Here's how the part is built. I have some questions about the finished solid (model axes, mm). A direction names the side the tool comes from. Round coordinates to 2 decimals unless told otherwise and drop trailing zeros. Loops run counter-clockwise (first coordinate to the right, second up) from the corner with the lowest first, then second, coordinate; pieces in that order, holes last. Notation, with made-up numbers: M 52.25,10.25 L 104.25,10.25 A17 ccw 104.25,33.25 Z; hole C 28,34.5 d2. An arc over 180 degrees is marked long. Use a Markdown table: item, result.
```python
from build123d import *

# Parameters (mm, degrees)
SKETCH2_R           = 41.5
SKETCH2_R_2         = 36.5
BOSS_EXTRUDE2_DEPTH = 140
BOSS_EXTRUDE3_START = -5
SKETCH13_R          = 41.5
SKETCH13_R_2        = 4.5
BOSS_EXTRUDE3_DEPTH = 5
CUT_EXTRUDE1_DEPTH  = 39
CUT_EXTRUDE2_DEPTH  = 39
CUT_EXTRUDE3_DEPTH  = 39
CUT_EXTRUDE4_DEPTH  = 39


with BuildPart() as part:
    # Sketch2 → Boss-Extrude2 (new body)
    with BuildSketch(Plane.XY):
        Circle(SKETCH2_R)
        Circle(SKETCH2_R_2, mode=Mode.SUBTRACT)
    extrude(amount=BOSS_EXTRUDE2_DEPTH)

    # Sketch13 → Boss-Extrude3 (add)
    with BuildSketch(Plane.XY.offset(BOSS_EXTRUDE3_START)):
        Circle(SKETCH13_R)
        Circle(SKETCH13_R_2, mode=Mode.SUBTRACT)
    extrude(amount=BOSS_EXTRUDE3_DEPTH)

    # Sketch14 → Cut-Extrude1 (cut)
    with BuildSketch(Plane(origin=(0, 0, 0), x_dir=(1, 0, 0), z_dir=(0, 1, 0))):
        Polygon((3.5, -127), (10.5, -127), (10.5, -122), (-3.5, -122), (-3.5, -140), (3.5, -140), align=None)
    extrude(amount=-CUT_EXTRUDE1_DEPTH, mode=Mode.SUBTRACT)

    # Sketch16 → Cut-Extrude2 (cut)
    with BuildSketch(Plane(origin=(0, 0, 0), x_dir=(0, 0, -1), z_dir=(1, 0, 0))):
        Polygon((-140, 3.548648678), (-127, 3.548648678), (-127, 10.548648678), (-122, 10.548648678), (-122, -3.451351322), (-140, -3.451351322), align=None)
    extrude(amount=CUT_EXTRUDE2_DEPTH, mode=Mode.SUBTRACT)

    # Sketch19 → Cut-Extrude3 (cut)
    with BuildSketch(Plane(origin=(0, 0, 0), x_dir=(1, 0, 0), z_dir=(0, 1, 0))):
        Polygon((3.5, -140), (3.5, -122), (-10.5, -122), (-10.5, -127), (-3.5, -127), (-3.5, -140), align=None)
    extrude(amount=CUT_EXTRUDE3_DEPTH, mode=Mode.SUBTRACT)

    # Sketch20 → Cut-Extrude4 (cut)
    with BuildSketch(Plane(origin=(0, 0, 0), x_dir=(0, 0, -1), z_dir=(1, 0, 0))):
        Polygon((-127, -3.5), (-140, -3.5), (-140, 3.5), (-122, 3.5), (-122, -10.5), (-127, -10.5), align=None)
    extrude(amount=-CUT_EXTRUDE4_DEPTH, mode=Mode.SUBTRACT)


solid = part.part
```
Q1. Will these pins go through, and if not, where does the flat tip stop? P1, Ø2, axis at x = -29, z = 95.5, coming from the -Y side; P2, Ø2, axis at y = 7, z = 94, coming from the +X side; P3, Ø6, axis at x = 16.5, y = -8, coming from the +Z side.
Return value:
| item | result |
|---|---|
| P1 | stops at y = -30.63 |
| P2 | stops at x = 41.06 |
| P3 | stops at z = 0 |
Q2. For faces 4 (the cylindrical face through (34.814, 10.964, 69.02)), 5 (the flat face through (-1, -9, -5)), 6 (the flat face through (10.5, -37, 125)), which set-ups out of +Z, -Z, +X, -X, +Y, -Y let a thin tool reach every point of the face, with its end or its side?
Return value:
| item | result |
|---|---|
| face 4 | +Z |
| face 5 | -Z, +X, -X, +Y, -Y |
| face 6 | none |
Q3. We'd pull the mould along X, two halves only. Please class faces 1 (the flat face through (24, 28, 140)), 2 (the flat face through (2, -39, 129)), 3 (the cylindrical face through (39.584, 12.465, 66.485)): pulls with the +X half, pulls with the -X half, needs draft (parallel to the pull), parting line crosses it, or undercut.
Return value:
| item | result |
|---|---|
| face 1 | needs draft |
| face 2 | undercut |
| face 3 | parting line crosses it |
Q4. I need wall thicknesses on line 1 (Y direction, x = 0, z = 67); line 2 (Z direction, x = 1, y = -5); line 3 (X direction, y = -24, z = 132.5). Which ranges of each line are inside material? Lowest first, please. Write a range as from..to.
Return value:
| item | result |
|---|---|
| line 1 | y = -41.5..-36.5, 36.5..41.5 |
| line 2 | z = -5..0 |
| line 3 | x = -33.86..-27.5, 27.5..33.86 |
Q5. Imagine slicing it at D-D, the plane y = -22.5. Please give me the cut outline in (x, z), then the cut area to 3 significant figures.
Return value:
| item | result |
|---|---|
| outline | M -34.87,-5 L 34.87,-5 L 34.87,140 L 28.74,140 L 28.74,0 L -28.74,0 L -28.74,140 L -34.87,140 Z |
| area | 2,070 mm^2 |
Q6. Imagine slicing it at A-A, the plane y = 0. Please give me the cut outline in (x, z), then the cut area to 3 significant figures.
Return value:
| item | result |
|---|---|
| outline | M -41.5,-5 L -4.5,-5 L -4.5,0 L -36.5,0 L -36.5,122 L -39,122 L -39,140 L -41.5,140 Z; M 4.5,-5 L 41.5,-5 L 41.5,140 L 39,140 L 39,122 L 36.5,122 L 36.5,0 L 4.5,0 Z |
| area | 1,680 mm^2 |
Q7. Imagine slicing it at C-C, the plane z = 35. Please give me the cut outline in (x, y).
Return value:
| item | result |
|---|---|
| outline | C 0,0 d83; hole C 0,0 d73 |
